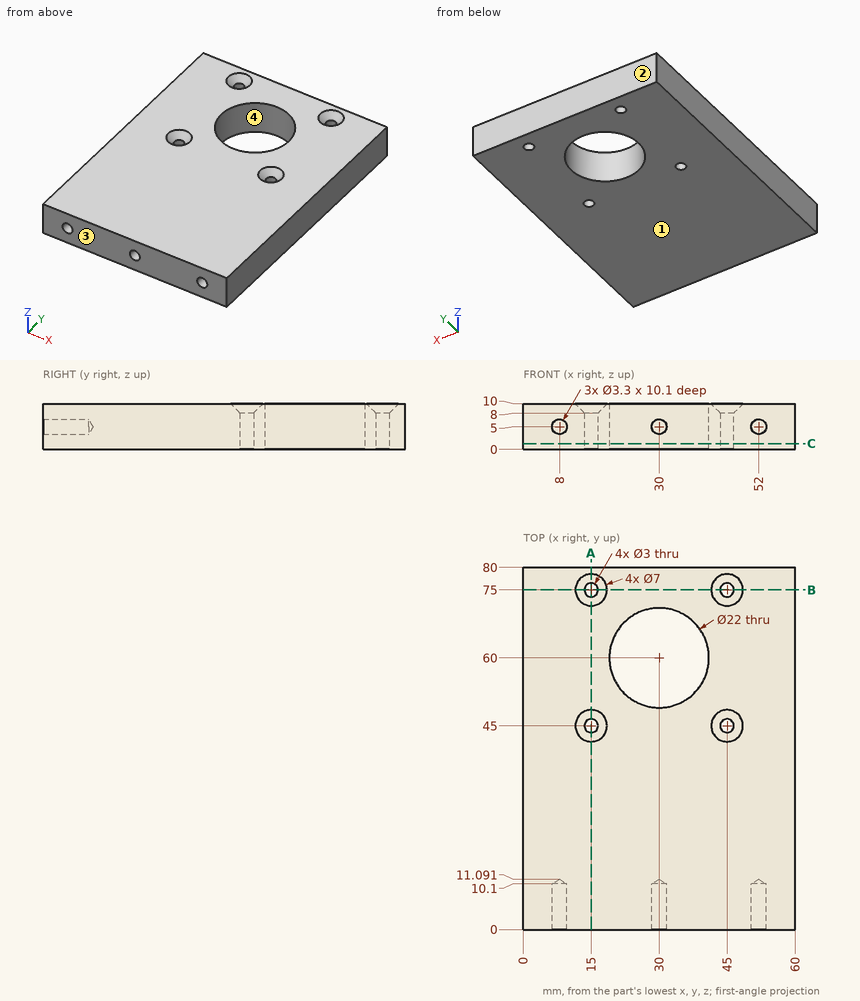
Geometry check sheet. Reference: drawing and pictorial views, mm from the part's lowest x, y, z. Round coordinates to 2 decimals unless told otherwise and drop trailing zeros. Loops run counter-clockwise (first coordinate to the right, second up) from the corner with the lowest first, then second, coordinate; pieces in that order, holes last. Notation, with made-up numbers: M -5.5,60.5 L 48.5,60.5 A26 ccw 48.5,82.5 Z; hole C 80,-14 d9. An arc over 180 degrees is marked long. One line per item, written item: value.
(1) Thickness scan on line 1 (Y direction, x = 15, z = 5.5); line 2 (X direction, y = 5.75, z = 5); line 3 (Z direction, x = 52, y = 5.5). Record the ranges inside material, lowest first.
Computed values:
line 1: y = 0 to 43.5, 46.5 to 73.5, 76.5 to 80
line 2: x = 0 to 6.35, 9.65 to 28.35, 31.65 to 50.35, 53.65 to 60
line 3: z = 0 to 3.35, 6.65 to 10
(2) Release check for a two-part mould opening along Y. For the marked faces 1, 2, 3 and 4 record: +Y half, -Y half, draft (parallel to the pull), parting line (faces both ways), or undercut.
Computed values:
face 1: draft
face 2: +Y half
face 3: -Y half
face 4: undercut
(3) Sectioned sample at B-B, the plane y = 75. Record the cut outline in (x, z), then the cut area to 3 significant figures.
Computed values:
outline: M 0,0 L 13.5,0 L 13.5,8 L 11.5,10 L 0,10 Z; M 16.5,0 L 43.5,0 L 43.5,8 L 41.5,10 L 18.5,10 L 16.5,8 Z; M 46.5,0 L 60,0 L 60,10 L 48.5,10 L 46.5,8 Z
area: 532 mm^2
(4) Depth check by flat-ended pin: pin 1 Ø3.5 at (x, y) = (45, 45) entering from +Z. Enter the tip coordinate at first touch or a pass-through.
Computed values:
pin 1: stops at z = 8.25
(5) Sectioned sample at C-C, the plane z = 1.25. Record the cut outline in (x, y), then the cut area to 3 significant figures.
Computed values:
outline: M 0,0 L 60,0 L 60,80 L 0,80 Z; hole C 15,45 d3; hole C 15,75 d3; hole C 30,60 d22; hole C 45,45 d3; hole C 45,75 d3
area: 4,390 mm^2
(6) Sectioned sample at A-A, the plane x = 15. Record the cut outline in (y, z).
Computed values:
outline: M 0,0 L 43.5,0 L 43.5,8 L 41.5,10 L 0,10 Z; M 46.5,0 L 73.5,0 L 73.5,8 L 71.5,10 L 48.5,10 L 46.5,8 Z; M 76.5,0 L 80,0 L 80,10 L 78.5,10 L 76.5,8 Z
